```python
from build123d import *

# Parameters (mm, degrees)
SKETCH1_W            = 466
SKETCH1_H            = 100
BOSS_EXTRUDE1_DEPTH  = 6
M8_CLEARANCE_SLOT1_D = 8.4
SKETCH4_W            = 25
SKETCH4_H            = 25
CUT_EXTRUDE1_DEPTH   = 12
SKETCH5_W            = 6
SKETCH5_H            = 12.5
CUT_EXTRUDE2_DEPTH   = 477.646619625


with BuildPart() as part:
    # Sketch1 → Boss-Extrude1 (new body)
    with BuildSketch(Plane.XY):
        with Locations((233, 50)):
            Rectangle(SKETCH1_W, SKETCH1_H)
    extrude(amount=BOSS_EXTRUDE1_DEPTH)

    # M8 Clearance Slot1 (through all)
    with Locations(Plane.XY.offset(6)):
        with Locations((24, 50), (442, 50)):
            Hole(M8_CLEARANCE_SLOT1_D / 2)

    # Sketch4 → Cut-Extrude1 (cut)
    with BuildSketch(Plane(origin=(0, 0, 0), x_dir=(-1, 0, 0), z_dir=(0, 0, -1))):
        with Locations((-87.5, 12.5)):
            Rectangle(SKETCH4_W, SKETCH4_H)
    extrude(amount=-CUT_EXTRUDE1_DEPTH, mode=Mode.SUBTRACT)

    # Sketch5 → Cut-Extrude2 (cut, through all)
    with BuildSketch(Plane(origin=(0, 0, 0), x_dir=(-1, 0, 0), z_dir=(0, 0, -1))):
        with Locations((-297, 93.75)):
            Rectangle(SKETCH5_W, SKETCH5_H)
        with Locations((-187, 93.75)):
            Rectangle(SKETCH5_W, SKETCH5_H)
        with Locations((-297, 6.25)):
            Rectangle(SKETCH5_W, SKETCH5_H)
        with Locations((-187, 6.25)):
            Rectangle(SKETCH5_W, SKETCH5_H)
    extrude(amount=-CUT_EXTRUDE2_DEPTH, mode=Mode.SUBTRACT)


solid = part.part
```
The listing builds one solid part. Answer for the finished solid, in the listing's coordinates (mm). Round coordinates to 2 decimals unless told otherwise and drop trailing zeros. Write each loop counter-clockwise with the first axis right and the second up, starting at its lowest first coordinate (ties: lowest second). Pieces come first, ordered by that corner, then holes. Notation, with made-up numbers: (69, 16.5) -> (124, 16.5) arc R24 cw to (124, 37.5) -> close; hole circle Ø6 at (-29, 71). An arc over 180 degrees is marked (long way). Answer as a JSON object with one key per item and string values. Group by question number.
Q1. Straight lines are drawn through the part: line 1 along X through (y, z) = (91, 1.2); line 2 along X through (y, z) = (17, 3.45); line 3 along Y through (x, z) = (442, 1.6). For each, find the intervals that lie inside material, in ascending order.
Q2. Determine the mould class of faces 1 (the face through (230, 51, 6)), 2 (the face through (446.196, 50.185, 2.958)), 3 (the face through (27.096, 52.839, 2.958)) for opening direction Y: pulls with the +Y half, pulls with the -Y half, needs draft (parallel to the pull), parting line crosses it, or undercut.
Q3. This flat-tipped pin is pushed along its axis until it touches: pin 1 Ø6.5 at (x, y) = (24, 50) entering from -Z. Where does it stop, or does it pass through?
Q4. Section A-A (y = 50) is taken. Write down the section's boundary in (x, z), plus the area to 3 significant figures.
Q5. Section C-C (z = 4.95) is taken. Write down the section's boundary in (x, y), plus the area to 3 significant figures.
Q6. Section B-B (x = 442) is taken. Write down the section's boundary in (y, z), plus the area to 3 significant figures.
Check values:
{
 "1": {"line 1": "0 to 184, 190 to 294, 300 to 466", "line 2": "0 to 75, 100 to 466", "line 3": "0 to 45.8, 54.2 to 100"},
 "2": {"face 1": "needs draft", "face 2": "undercut", "face 3": "undercut"},
 "3": {"pin 1": "through"},
 "4": {"outline": "(0, 0) -> (19.8, 0) -> (19.8, 6) -> (0, 6) -> close; (28.2, 0) -> (437.8, 0) -> (437.8, 6) -> (28.2, 6) -> close; (446.2, 0) -> (466, 0) -> (466, 6) -> (446.2, 6) -> close", "area": "2,700 mm^2"},
 "5": {"outline": "(0, 0) -> (75, 0) -> (75, 25) -> (100, 25) -> (100, 0) -> (184, 0) -> (184, 12.5) -> (190, 12.5) -> (190, 0) -> (294, 0) -> (294, 12.5) -> (300, 12.5) -> (300, 0) -> (466, 0) -> (466, 100) -> (300, 100) -> (300, 87.5) -> (294, 87.5) -> (294, 100) -> (190, 100) -> (190, 87.5) -> (184, 87.5) -> (184, 100) -> (0, 100) -> close; hole circle Ø8.4 at (24, 50); hole circle Ø8.4 at (442, 50)", "area": "45,600 mm^2"},
 "6": {"outline": "(0, 0) -> (45.8, 0) -> (45.8, 6) -> (0, 6) -> close; (54.2, 0) -> (100, 0) -> (100, 6) -> (54.2, 6) -> close", "area": "550 mm^2"}
}
